Can you work these out from the model? Positions are in its coordinate system, mm. Round coordinates to 2 decimals unless told otherwise and drop trailing zeros. Order: outer loops, then holes, each group sorted by start corner. A loop starts at its lowest first (then second) coordinate and runs counter-clockwise, first axis right, second up. Notation, with made-up numbers: (35.25, 76) - (60.25, 76) arc R25 ccw to (60.25, 93) - close; hole circle Ø11 at (-30, -11.75). An arc over 180 degrees is marked (long way). Write item = value, one per line.
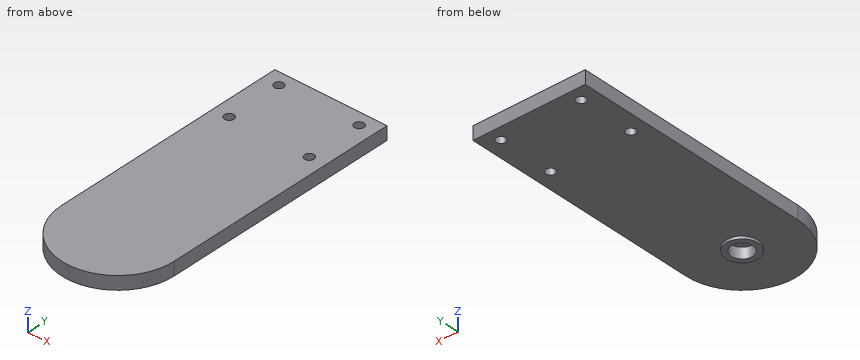
from build123d import *

# Parameters (mm, degrees)
BOSS_EXTRUDE1_DEPTH = 5
SKETCH2_R           = 1.75
CUT_EXTRUDE1_DEPTH  = 93.552687697
SKETCH3_R           = 4
CUT_EXTRUDE2_DEPTH  = 3
BOSS_EXTRUDE2_START = 1
SKETCH4_R           = 6
SKETCH4_R_2         = 4
BOSS_EXTRUDE2_DEPTH = 1


with BuildPart() as part:
    # Sketch1 → Boss-Extrude1 (new body)
    with BuildSketch(Plane.XY):
        with BuildLine():
            Line((-21, 0), (-21, 90))
            Line((-21, 90), (21, 90))
            Line((21, 90), (21, 0))
            ThreePointArc((21, 0), (0, -21), (-21, 0))
        make_face()
    extrude(amount=BOSS_EXTRUDE1_DEPTH)

    # Sketch2 → Cut-Extrude1 (cut, through all)
    with BuildSketch(Plane(origin=(0, 0, 0), x_dir=(-1, 0, 0), z_dir=(0, 0, -1))):
        with Locations((-15, 85)):
            Circle(SKETCH2_R)
        with Locations((-15, 64)):
            Circle(SKETCH2_R)
        with Locations(Location((15, 64, 0), (0, 0, 180))):
            Circle(SKETCH2_R)
        with Locations(Location((15, 85, 0), (0, 0, 180))):
            Circle(SKETCH2_R)
    extrude(amount=-CUT_EXTRUDE1_DEPTH, mode=Mode.SUBTRACT)

    # Sketch3 → Cut-Extrude2 (cut)
    with BuildSketch(Plane(origin=(0, 0, 0), x_dir=(-1, 0, 0), z_dir=(0, 0, -1))):
        Circle(SKETCH3_R)
    extrude(amount=-CUT_EXTRUDE2_DEPTH, mode=Mode.SUBTRACT)

    # Sketch4 → Boss-Extrude2 (add)
    with BuildSketch(Plane(origin=(0, 0, 0), x_dir=(-1, 0, 0), z_dir=(0, 0, -1)).offset(BOSS_EXTRUDE2_START)):
        with Locations(Location((0, 0, 0), (0, 0, 180))):
            Circle(SKETCH4_R)
        Circle(SKETCH4_R_2, mode=Mode.SUBTRACT)
    extrude(amount=-BOSS_EXTRUDE2_DEPTH)


solid = part.part
(1) If we section it at B-B (x = 15): Write out the boundary of the cut face in (y, z).
Computed:
outline = (-14.7, 0) - (62.25, 0) - (62.25, 5) - (-14.7, 5) - close; (65.75, 0) - (83.25, 0) - (83.25, 5) - (65.75, 5) - close; (86.75, 0) - (90, 0) - (90, 5) - (86.75, 5) - close
(2) If we section it at C-C (z = 4.1): Write out the boundary of the cut face in (x, y).
Computed:
outline = (-21, 0) arc R21 ccw to (21, 0) - (21, 90) - (-21, 90) - close; hole circle Ø3.5 at (-15, 64); hole circle Ø3.5 at (-15, 85); hole circle Ø3.5 at (15, 64); hole circle Ø3.5 at (15, 85)
(3) Will these pins go through, and if not, where does the flat tip stop? P1, Ø5.5, axis at x = -15, y = 64, coming from the -Z side; P2, Ø3, axis at x = 15, y = 85, coming from the +Z side; P3, Ø1, axis at x = -3, z = 0.5, coming from the -Y side; P4, Ø1.5, axis at x = -4.5, z = 1, coming from the -Y side.
Computed:
P1 = 0
P2 = through
P3 = -20.85
P4 = -20.66
(4) If I drill on line 1 (X direction, y = 64, z = 2.7); line 2 (Y direction, x = -15, z = 2.15); line 3 (Y direction, x = -15.5, z = 4.15), over which ranges is the centre line in solid material (lowest first)? Write a range as from..to.
Computed:
line_1 = -21..-16.75, -13.25..13.25, 16.75..21
line_2 = -14.7..62.25, 65.75..83.25, 86.75..90
line_3 = -14.17..62.32, 65.68..83.32, 86.68..90
(5) If we section it at D-D (x = 0.5): Write out the boundary of the cut face in (y, z).
Computed:
outline = (-20.99, 0) - (-5.98, 0) - (-5.98, -1) - (-3.97, -1) - (-3.97, 3) - (3.97, 3) - (3.97, -1) - (5.98, -1) - (5.98, 0) - (90, 0) - (90, 5) - (-20.99, 5) - close
(6) If we section it at A-A (y = 64): Write out the boundary of the cut face in (x, z), plus the area to 3 significant figures.
Computed:
outline = (-21, 0) - (-16.75, 0) - (-16.75, 5) - (-21, 5) - close; (-13.25, 0) - (13.25, 0) - (13.25, 5) - (-13.25, 5) - close; (16.75, 0) - (21, 0) - (21, 5) - (16.75, 5) - close
area = 175 mm^2
